The drawing under review shows one solid part. Ordinate dimensions are in mm from its lowest x, y, z. Coordinates: 2 decimals unless noted, no trailing zeros. Loops run counter-clockwise (first coordinate to the right, second up) from the corner with the lowest first, then second, coordinate; pieces in that order, holes last. Notation, with made-up numbers: M 34,-18.75 L 73,-18.75 A32 cw 73,17.25 Z; hole C 13.5,-7.5 d10. An arc over 180 degrees is marked long. Use one line per item in the form item = value.
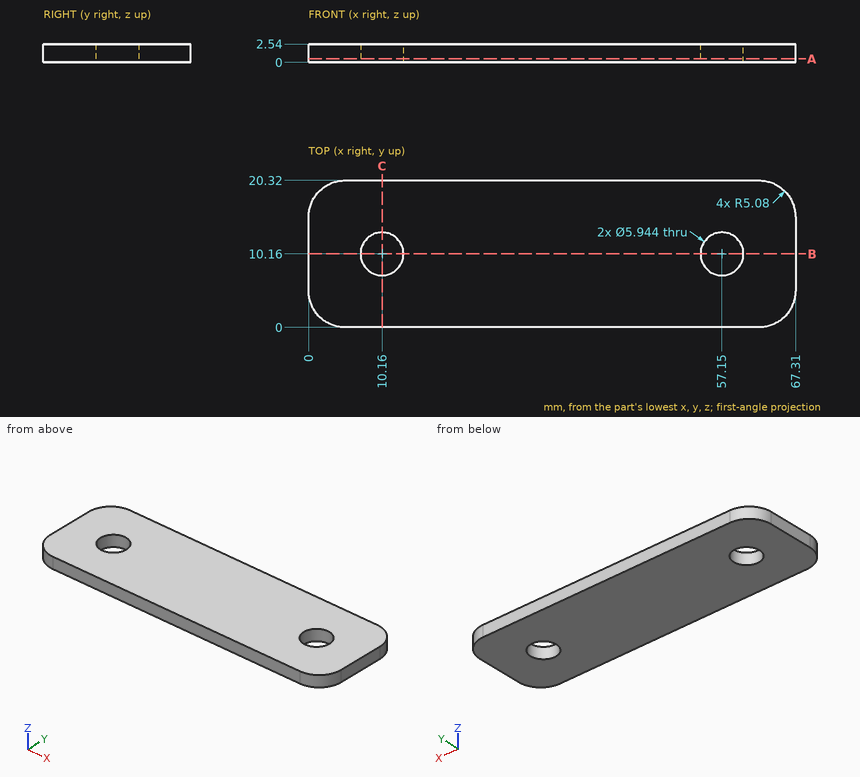
1. Consider section B-B on y = 10.16. Write out the cut boundary in (x, z).
Computed values:
outline = M 0,0 L 7.19,0 L 7.19,2.54 L 0,2.54 Z; M 13.13,0 L 54.18,0 L 54.18,2.54 L 13.13,2.54 Z; M 60.12,0 L 67.31,0 L 67.31,2.54 L 60.12,2.54 Z
2. Consider section C-C on x = 10.16. Write out the cut boundary in (y, z), plus the area to 3 significant figures.
Computed values:
outline = M 0,0 L 7.19,0 L 7.19,2.54 L 0,2.54 Z; M 13.13,0 L 20.32,0 L 20.32,2.54 L 13.13,2.54 Z
area = 36.5 mm2
3. For pin 1 Ø1 at (x, y) = (20.5, 4.5) entering from -Z; pin 2 Ø5.5 at (x, y) = (57.15, 10.16) entering from -Z, all flat-tipped, find the tip position at first contact; note any pin that passes through.
Computed values:
pin_1 = 0
pin_2 = through
4. Wall thickness on line 1 along X through (y, z) = (8.75, 0.8) (1 decimal); line 2 along Y through (x, z) = (10.16, 1.1); line 3 along X through (y, z) = (8.25, 1.75) (1 decimal): over which ranges is each line inside the solid? List them lowest first. Write a range as from..to.
Computed values:
line_1 = 0..7.5, 12.8..54.5, 59.8..67.3
line_2 = 0..7.19, 13.13..20.32
line_3 = 0..7.9, 12.4..54.9, 59.4..67.3
5. Consider section A-A on z = 0.5. Write out the cut boundary in (x, y), plus the area to 3 significant figures.
Computed values:
outline = M 0,5.08 A5.08 ccw 5.08,0 L 62.23,0 A5.08 ccw 67.31,5.08 L 67.31,15.24 A5.08 ccw 62.23,20.32 L 5.08,20.32 A5.08 ccw 0,15.24 Z; hole C 10.16,10.16 d5.94; hole C 57.15,10.16 d5.94
area = 1,290 mm2
